from build123d import *

# Parameters (mm, degrees)
BOSS_EXTRUDE1_DEPTH = 5
SKETCH2_R           = 2.55
CUT_EXTRUDE1_DEPTH  = 10
CHAMFER1_SIZE       = 10
CHAMFER2_SIZE       = 4
CHAMFER3_SIZE       = 4


with BuildPart() as part:
    # Sketch1 → Boss-Extrude1 (new body)
    with BuildSketch(Plane.XY):
        Polygon((0, 0), (0, 80), (20, 80), (20, 40), (40, 40), (40, 0), align=None)
    extrude(amount=BOSS_EXTRUDE1_DEPTH)

    # Sketch2 → Cut-Extrude1 (cut)
    with BuildSketch(Plane.XY.offset(5)):
        with Locations((10, 70)):
            Circle(SKETCH2_R)
        with Locations((10, 50)):
            Circle(SKETCH2_R)
        with Locations((10, 30)):
            Circle(SKETCH2_R)
        with Locations((10, 10)):
            Circle(SKETCH2_R)
        with Locations((30, 30)):
            Circle(SKETCH2_R)
        with Locations((30, 10)):
            Circle(SKETCH2_R)
    extrude(amount=-CUT_EXTRUDE1_DEPTH, mode=Mode.SUBTRACT)

    # Chamfer1
    chamfer1_edges = [part.edges().sort_by_distance(p)[0] for p in [
        (20, 40, 2.5),
    ]]
    chamfer(chamfer1_edges, length=CHAMFER1_SIZE)

    # Chamfer2
    chamfer2_edges = [part.edges().sort_by_distance(p)[0] for p in [
        (20, 80, 2.5),
    ]]
    chamfer(chamfer2_edges, length=CHAMFER2_SIZE)

    # Chamfer3
    chamfer3_edges = [part.edges().sort_by_distance(p)[0] for p in [
        (0, 0, 2.5),
        (0, 80, 2.5),
        (40, 40, 2.5),
        (40, 0, 2.5),
    ]]
    chamfer(chamfer3_edges, length=CHAMFER3_SIZE)


solid = part.part
Here's how the part is built. I have some questions about the finished solid (model axes, mm). A direction names the side the tool comes from. Coordinates: 2 decimals unless noted, no trailing zeros. Write each loop counter-clockwise with the first axis right and the second up, starting at its lowest first coordinate (ties: lowest second). Pieces come first, ordered by that corner, then holes.
1) If we section it at A-A (z = 1.95): List the corners of the cut face in (x, y) for me, plus the area to 3 significant figures.
Filled in:
outline: (0, 4) - (4, 0) - (36, 0) - (40, 4) - (40, 36) - (36, 40) - (30, 40) - (20, 50) - (20, 76) - (16, 80) - (4, 80) - (0, 76) - close; hole circle Ø5.1 at (10, 10); hole circle Ø5.1 at (10, 30); hole circle Ø5.1 at (10, 50); hole circle Ø5.1 at (10, 70); hole circle Ø5.1 at (30, 10); hole circle Ø5.1 at (30, 30)
area: 2,290 mm2
2) If we section it at D-D (y = 38.5): List the corners of the cut face in (x, z) for me.
Filled in:
outline: (0, 0) - (37.5, 0) - (37.5, 5) - (0, 5) - close
3) If we section it at B-B (y = 70): List the corners of the cut face in (x, z) for me, plus the area to 3 significant figures.
Filled in:
outline: (0, 0) - (7.45, 0) - (7.45, 5) - (0, 5) - close; (12.55, 0) - (20, 0) - (20, 5) - (12.55, 5) - close
area: 74.5 mm2
4) Which directions (+Z, -Z, +X, -X, +Y, -Y) give clear straight access to the entire face, cutting with the end or side of a thin tool? Please do faces 5 (the face through (38, 2, 2)), 6 (the face through (33, 40, 2)).
Filled in:
face 5: +Z, -Z, +X, -Y
face 6: +Z, -Z, +X, +Y
5) Thinking about a two-plate mould opening in X: for faces 1 (the face through (2, 78, 2)), 2 (the face through (10, 80, 2)), 3 (the face through (9.67, 52.53, 2.54)), 4 (the face through (28.1, 31.7, 2.5)), which applies, +X half, -X half, draft (parallel to the pull), parting line (faces both ways), or undercut?
Filled in:
face 1: -X half
face 2: draft
face 3: undercut
face 4: undercut
6) I'm going to push a flat-ended pin straight in: pin 1 (1 mm diameter, centred on x = 35.5, z = 3.5, fed in from +Y). Where does the tip first touch, or does it pass through?
Filled in:
pin 1: stops at y = 40
7) If we section it at C-C (y = 10): List the corners of the cut face in (x, z) for me.
Filled in:
outline: (0, 0) - (7.45, 0) - (7.45, 5) - (0, 5) - close; (12.55, 0) - (27.45, 0) - (27.45, 5) - (12.55, 5) - close; (32.55, 0) - (40, 0) - (40, 5) - (32.55, 5) - close
8) If I drill on line 1 (Y direction, x = 30, z = 3.3); line 2 (Y direction, x = 10, z = 2.35); line 3 (Y direction, x = 9, z = 2.1), over which ranges is the centre line in solid material (lowest first)?
Filled in:
line 1: y = 0 to 7.45, 12.55 to 27.45, 32.55 to 40
line 2: y = 0 to 7.45, 12.55 to 27.45, 32.55 to 47.45, 52.55 to 67.45, 72.55 to 80
line 3: y = 0 to 7.65, 12.35 to 27.65, 32.35 to 47.65, 52.35 to 67.65, 72.35 to 80
